Geometry check sheet. Reference: drawing and pictorial views, mm from the part's lowest x, y, z. A direction names the side the tool comes from. Coordinates: 2 decimals unless noted, no trailing zeros. Write each loop counter-clockwise with the first axis right and the second up, starting at its lowest first coordinate (ties: lowest second). Pieces come first, ordered by that corner, then holes. Notation, with made-up numbers: M 34.25,31.25 L 88.25,31.25 A15 ccw 88.25,60.25 Z; hole C 12,74.5 d5. An arc over 180 degrees is marked long. One line per item, written item: value.
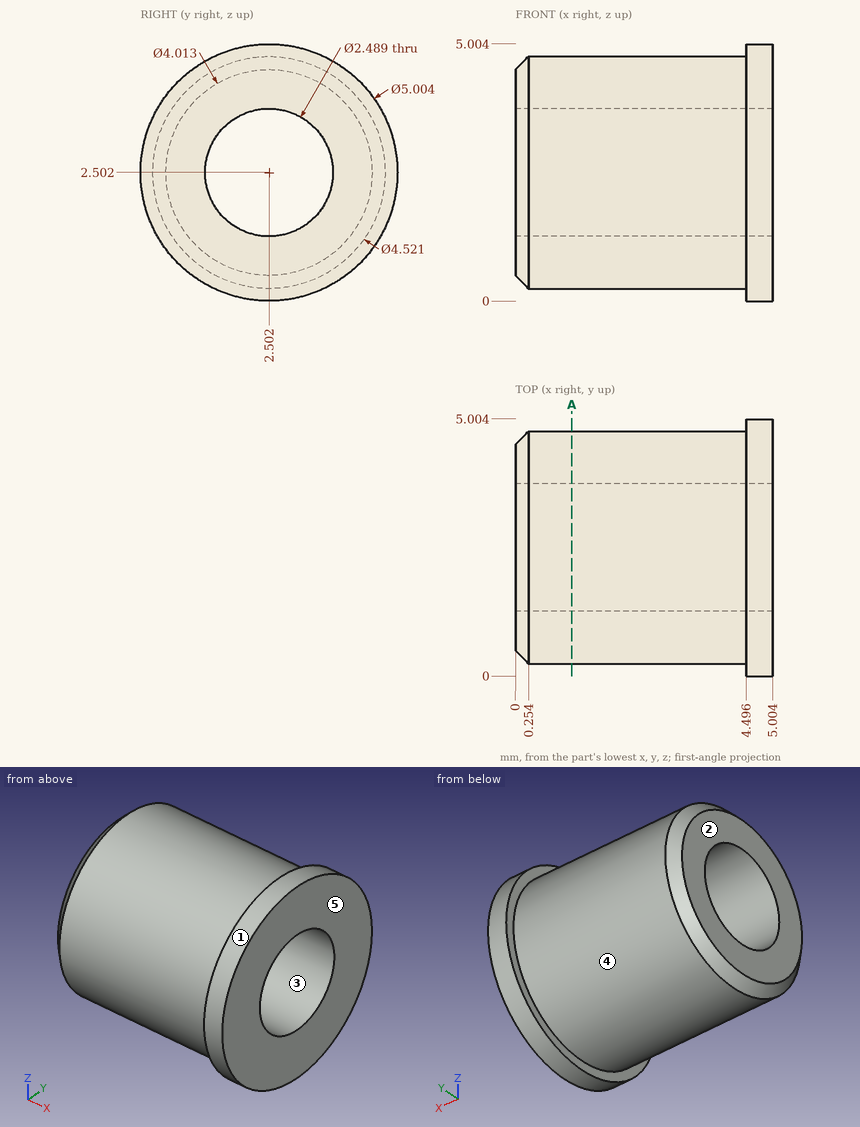
Item 1: Draft check along Z on the marked faces 1, 2 and 3. Enter one of: released by +Z, released by -Z, zero draft, split by the parting line, or undercut.
The answers:
face 1: split by the parting line
face 2: zero draft
face 3: undercut
Item 2: Go/stop test with flat-tipped pins: P1, Ø1.5, axis at x = 2.5, y = 1.5, coming from the -Z side; P2, Ø1, axis at x = 0.5, y = 2, coming from the -Z side. Record where each tip stops, or that it passes through.
The answers:
P1: stops at z = 0.26
P2: stops at z = 0.24
Item 3: Scan lines: line 1 (X direction, y = 1.6, z = 4.65); line 2 (Z direction, x = 1.65, y = 3.1); line 3 (Y direction, x = 4.4, z = 1.5) (1 decimal). Record each from-to range of solid material in increasing order.
The answers:
line 1: x = 4.5 to 5
line 2: z = 0.32 to 1.41, 3.59 to 4.68
line 3: y = 0.5 to 1.8, 3.2 to 4.5
Item 4: Access from +Z, -Z, +X, -X, +Y, -Y to the whole of each face (thin tool, end or side, straight path). Record for the marked faces 4 and 5.
The answers:
face 4: -X
face 5: +Z, -Z, +X, +Y, -Y
Item 5: Cross-section at A-A, the plane x = 1.1. Enter the section's corners in (y, z) (1 decimal), and give its area (3 significant figures).
The answers:
outline: C 2.5,2.5 d4.5; hole C 2.5,2.5 d2.5
area: 11.2 mm²
